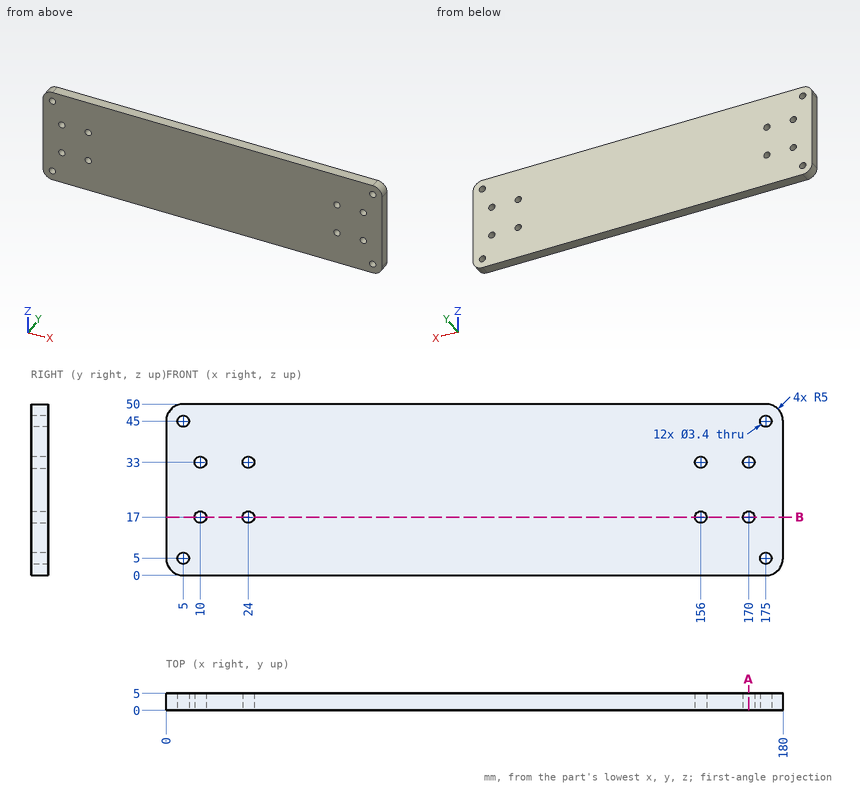
Geometry check sheet. Reference: drawing and pictorial views, mm from the part's lowest x, y, z. Round coordinates to 2 decimals unless told otherwise and drop trailing zeros. Order: outer loops, then holes, each group sorted by start corner. A loop starts at its lowest first (then second) coordinate and runs counter-clockwise, first axis right, second up. Notation, with made-up numbers: M 47,26 L 74,26 A6 ccw 74,32 Z; hole C 71.5,39 d2. An arc over 180 degrees is marked long. Answer in a Markdown table with one row per item.
(1) Go/stop test with a flat-tipped pin: P1, Ø4.5, axis at x = 156, z = 33, coming from the +Y side. Record where the tip stops, or that it passes through.
Responses:
| item | result |
|---|---|
| P1 | stops at y = 5 |
(2) Sectioned sample at A-A, the plane x = 170. Record the cut outline in (y, z).
Responses:
| item | result |
|---|---|
| outline | M 0,0 L 5,0 L 5,15.3 L 0,15.3 Z; M 0,18.7 L 5,18.7 L 5,31.3 L 0,31.3 Z; M 0,34.7 L 5,34.7 L 5,50 L 0,50 Z |
(3) Sectioned sample at B-B, the plane z = 17. Record the cut outline in (x, y).
Responses:
| item | result |
|---|---|
| outline | M 0,0 L 8.3,0 L 8.3,5 L 0,5 Z; M 11.7,0 L 22.3,0 L 22.3,5 L 11.7,5 Z; M 25.7,0 L 154.3,0 L 154.3,5 L 25.7,5 Z; M 157.7,0 L 168.3,0 L 168.3,5 L 157.7,5 Z; M 171.7,0 L 180,0 L 180,5 L 171.7,5 Z |
(4) Scan lines: probe 1 along Z at (x, y) = (5, 3.6); probe 2 along X at (y, z) = (2.65, 33); probe 3 along Z at (x, y) = (24, 2.15). Record each from-to range of solid material in increasing order. Write a range as from..to.
Responses:
| item | result |
|---|---|
| probe 1 | z = 0..3.3, 6.7..43.3, 46.7..50 |
| probe 2 | x = 0..8.3, 11.7..22.3, 25.7..154.3, 157.7..168.3, 171.7..180 |
| probe 3 | z = 0..15.3, 18.7..31.3, 34.7..50 |
